Source: three-view drawing plus pictorial views. Frame: mm from the lowest corner of the part. Round coordinates to 2 decimals unless told otherwise and drop trailing zeros. Write each loop counter-clockwise with the first axis right and the second up, starting at its lowest first coordinate (ties: lowest second). Pieces come first, ordered by that corner, then holes. Notation, with made-up numbers: M -26.75,-7 L -6.75,-7 A13 cw -6.75,11 Z; hole C 12.5,47 d3. An arc over 180 degrees is marked long. Answer in a Markdown table with one row per item.
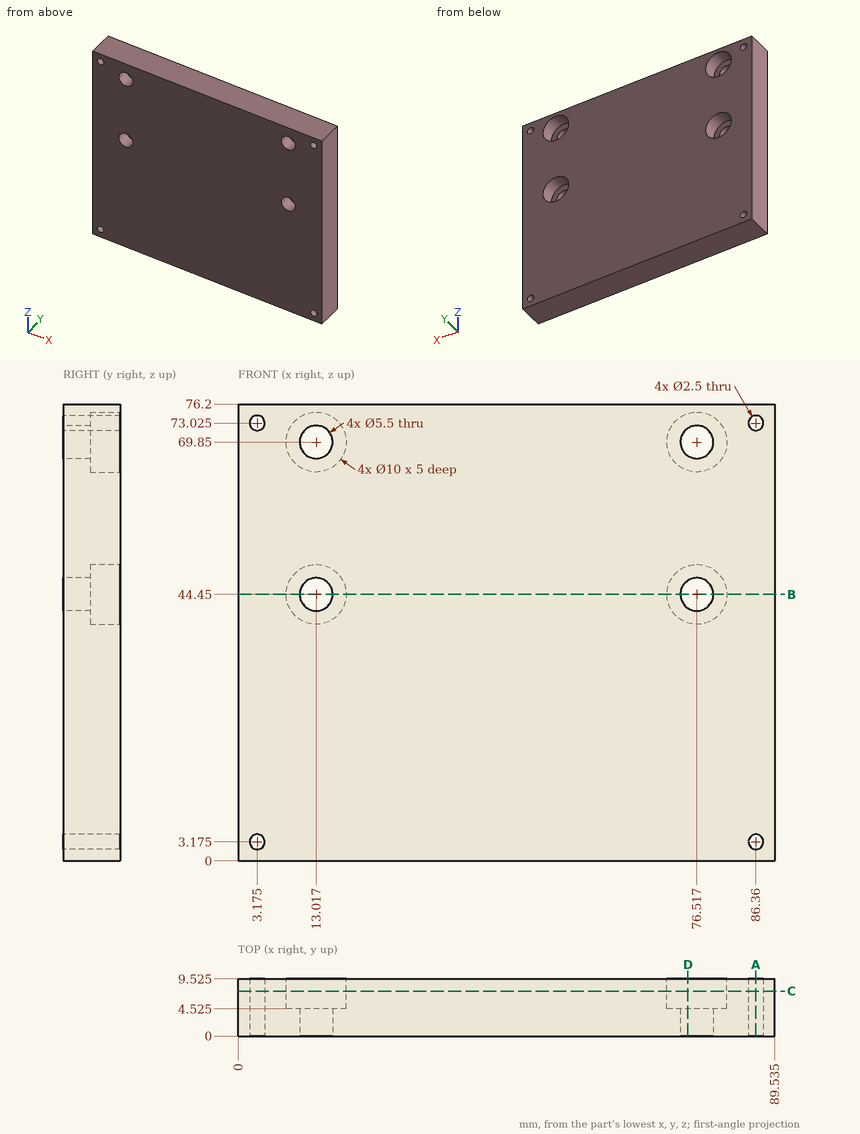
Q1. Section A-A (x = 86.36). Return loops of the section in (y, z) (1 decimal), and give its area (3 significant figures).
Solutions:
| item | result |
|---|---|
| outline | M 0,0 L 9.5,0 L 9.5,1.9 L 0,1.9 Z; M 0,4.4 L 9.5,4.4 L 9.5,71.8 L 0,71.8 Z; M 0,74.3 L 9.5,74.3 L 9.5,76.2 L 0,76.2 Z |
| area | 678 mm2 |
Q2. Section D-D (x = 75). Return loops of the section in (y, z) (1 decimal).
Solutions:
| item | result |
|---|---|
| outline | M 0,0 L 9.5,0 L 9.5,39.7 L 4.5,39.7 L 4.5,42.2 L 0,42.2 Z; M 0,46.7 L 4.5,46.7 L 4.5,49.2 L 9.5,49.2 L 9.5,65.1 L 4.5,65.1 L 4.5,67.6 L 0,67.6 Z; M 0,72.1 L 4.5,72.1 L 4.5,74.6 L 9.5,74.6 L 9.5,76.2 L 0,76.2 Z |
Q3. Section C-C (y = 7.5). State how many separate pieces and enclosed holes the cut face has, and give its area (3 significant figures).
Solutions:
| item | result |
|---|---|
| separate pieces | 1 |
| enclosed holes | 8 |
| area | 6,490 mm2 |
Q4. Section B-B (z = 44.45). Return loops of the section in (x, y) (1 decimal).
Solutions:
| item | result |
|---|---|
| outline | M 0,0 L 10.3,0 L 10.3,4.5 L 8,4.5 L 8,9.5 L 0,9.5 Z; M 15.8,0 L 73.8,0 L 73.8,4.5 L 71.5,4.5 L 71.5,9.5 L 18,9.5 L 18,4.5 L 15.8,4.5 Z; M 79.3,0 L 89.5,0 L 89.5,9.5 L 81.5,9.5 L 81.5,4.5 L 79.3,4.5 Z |
Q5. Material intervals for probe 1 along X at (y, z) = (7.45, 69.85) (1 decimal); probe 2 along Z at (x, y) = (86.5, 6); probe 3 along X at (y, z) = (3, 71) (1 decimal), sorted ascending.
Solutions:
| item | result |
|---|---|
| probe 1 | x = 0 to 8, 18 to 71.5, 81.5 to 89.5 |
| probe 2 | z = 0 to 1.93, 4.42 to 71.78, 74.27 to 76.2 |
| probe 3 | x = 0 to 10.5, 15.5 to 74, 79 to 89.5 |
Q6. Contact query for flat-ended pins moving along their axis: pin 1 Ø6.5 at (x, z) = (76.52, 69.85) entering from +Y (1 decimal); pin 2 Ø4.5 at (x, z) = (76.52, 44.45) entering from -Y. Output: stop coordinate, or through.
Solutions:
| item | result |
|---|---|
| pin 1 | stops at y = 4.5 |
| pin 2 | passes through |
